from build123d import *

# Parameters (mm, degrees)
SKETCH1_R                  = 1.85
SKETCH1_R_2                = 4
BOSS_EXTRUDE1_DEPTH        = 2
BOSS_EXTRUDE3_DEPTH        = 10
SKETCH12_R                 = 1.36525
CUT_EXTRUDE2_DEPTH         = 3
SKETCH14_R                 = 1.35255
CUT_EXTRUDE3_DEPTH         = 6
FILLET1_R                  = 10
FLATTEN_BENDS1_START       = 2
FLATTEN_BENDS1_DEPTH       = 10
FLATTEN_BENDS1_2_OUTLINE_R = 1.36525
FLATTEN_BENDS1_2_DEPTH     = 2
PROCESS_BENDS1_START       = -8.401979777
PROCESS_BENDS1_OUTLINE_W   = 29
PROCESS_BENDS1_OUTLINE_H   = 2
PROCESS_BENDS1_DEPTH       = 8.701769682
PROCESS_BENDS1_START_2     = 0.591569905
PROCESS_BENDS1_2_OUTLINE_W = 29
PROCESS_BENDS1_2_OUTLINE_H = 10
PROCESS_BENDS1_2_OUTLINE_R = 1.36525
PROCESS_BENDS1_2_DEPTH     = 1.70822
PROCESS_BENDS1_START_3     = 0.299789905
PROCESS_BENDS1_3_OUTLINE_W = 29
PROCESS_BENDS1_3_OUTLINE_H = 10
PROCESS_BENDS1_3_OUTLINE_R = 1.36525
PROCESS_BENDS1_3_DEPTH     = 3
PROCESS_BENDS1_START_4     = -6.292093187
PROCESS_BENDS1_4_DEPTH     = 29


with BuildPart() as part:
    # Sketch1 → Boss-Extrude1 (new body)
    with BuildSketch(Plane(origin=(0, 2, 0), x_dir=(1, 0, 0), z_dir=(0, 1, 0))):
        with BuildLine():
            Line((16.268898369, 15.844931419), (-4.237198285, -4.661165235))
            Line((-4.237198285, -4.661165235), (7.60163648, -16.5))
            Line((7.60163648, -16.5), (48.167251499, -16.5))
            Line((48.167251499, -16.5), (66.344250399, -13.294904666))
            ThreePointArc((66.344250399, -13.294904666), (77.499939542, -0.040402458), (66.423785357, 13.280634945))
            ThreePointArc((66.423785357, 13.280634945), (42.528480772, 15.498562339), (18.613829789, 13.5))
            Line((18.613829789, 13.5), (16.268898369, 15.844931419))
        make_face()
        with Locations(Location((56, 0, 0), (0, 0, 90))):
            Circle(SKETCH1_R, mode=Mode.SUBTRACT)
        with Locations(Location((64, -8, 0), (0, 0, 90))):
            Circle(SKETCH1_R, mode=Mode.SUBTRACT)
        with Locations(Location((72, 0, 0), (0, 0, 90))):
            Circle(SKETCH1_R, mode=Mode.SUBTRACT)
        with Locations(Location((64, 8, 0), (0, 0, 90))):
            Circle(SKETCH1_R, mode=Mode.SUBTRACT)
        with Locations(Location((64, 0, 0), (0, 0, 90))):
            Circle(SKETCH1_R_2, mode=Mode.SUBTRACT)
    extrude(amount=-BOSS_EXTRUDE1_DEPTH)

    # Sketch5 → Boss-Extrude3 (add)
    with BuildSketch(Plane(origin=(0, 2, 0), x_dir=(1, 0, 0), z_dir=(0, 1, 0))):
        Polygon((16.268898369, 15.844931419), (-4.237198285, -4.661165235), (-2.822984723, -6.075378798), (17.683111932, 14.430717857), align=None)
    extrude(amount=BOSS_EXTRUDE3_DEPTH)

    # Sketch12 → Cut-Extrude2 (cut)
    with BuildSketch(Plane(origin=(0.211983475, 0, 0.211983475), x_dir=(-0.7071067811865475, 0, 0.7071067811865477), z_dir=(-0.7071067811865477, 0, -0.7071067811865475))):
        with Locations((-16.207906813, 8)):
            Circle(SKETCH12_R)
        with Locations((-0.207906813, 8)):
            Circle(SKETCH12_R)
    extrude(amount=-CUT_EXTRUDE2_DEPTH, mode=Mode.SUBTRACT)

    # Sketch14 → Cut-Extrude3 (cut)
    with BuildSketch(Plane(origin=(0, 0, 0), x_dir=(1, 0, 0), z_dir=(0, 1, 0))):
        with Locations(Location((39.946755384, 11.867587507, 0), (0, 0, 270))):
            Circle(SKETCH14_R)
    extrude(amount=CUT_EXTRUDE3_DEPTH, mode=Mode.SUBTRACT)

    # Fillet1
    fillet1_edges = [part.edges().sort_by_distance(p)[0] for p in [
        (7.60163648, 1, 16.5),
    ]]
    fillet(fillet1_edges, radius=FILLET1_R)

    # Flatten-Bends1: read off the stored shape, not the designer's step
    # Flatten-Bends1 outline → Flatten-Bends1 (cut)
    with BuildSketch(Plane(origin=(0, 0, 0), x_dir=(1, 0, 0), z_dir=(0, 1, 0)).offset(FLATTEN_BENDS1_START)):
        Polygon((17.683111932, 14.430717857), (16.479779049, 15.634050739), (16.268898369, 15.844931419), (-4.237198285, -4.661165235), (-4.026317605, -4.872045915), (-2.822984722, -6.075378798), align=None)
    extrude(amount=FLATTEN_BENDS1_DEPTH, mode=Mode.SUBTRACT)

    # Flatten-Bends1 2 outline → Flatten-Bends1 2 (add)
    with BuildSketch(Plane(origin=(0, 0, 0), x_dir=(1, 0, 0), z_dir=(0, 1, 0))):
        Polygon((-4.237198285, -4.661165235), (16.268898369, 15.844931419), (10.115818019, 21.99801177), (-10.390278636, 1.491915115), align=None)
        with Locations((-2.965657433, 3.259682068)):
            Circle(FLATTEN_BENDS1_2_OUTLINE_R, mode=Mode.SUBTRACT)
        with Locations((8.348051066, 14.573390567)):
            Circle(FLATTEN_BENDS1_2_OUTLINE_R, mode=Mode.SUBTRACT)
    extrude(amount=FLATTEN_BENDS1_2_DEPTH)

    # Process-Bends1: read off the stored shape, not the designer's step
    # Process-Bends1 outline → Process-Bends1 (cut)
    with BuildSketch(Plane(origin=(0, 0, 0), x_dir=(0.7071067811865471, 0, -0.707106781186548), z_dir=(0.707106781186548, 0, 0.707106781186547)).offset(PROCESS_BENDS1_START)):
        with Locations((8.207906813, 1)):
            Rectangle(PROCESS_BENDS1_OUTLINE_W, PROCESS_BENDS1_OUTLINE_H)
    extrude(amount=PROCESS_BENDS1_DEPTH, mode=Mode.SUBTRACT)

    # Process-Bends1 2 outline → Process-Bends1 2 (add)
    with BuildSketch(Plane(origin=(0, 0, 0), x_dir=(0.7071067811865471, 0, -0.707106781186548), z_dir=(0.707106781186548, 0, 0.707106781186547)).offset(PROCESS_BENDS1_START_2)):
        with Locations((8.207906813, 7)):
            Rectangle(PROCESS_BENDS1_2_OUTLINE_W, PROCESS_BENDS1_2_OUTLINE_H)
        with Locations((0.207906813, 8)):
            Circle(PROCESS_BENDS1_2_OUTLINE_R, mode=Mode.SUBTRACT)
        with Locations((16.207906813, 8)):
            Circle(PROCESS_BENDS1_2_OUTLINE_R, mode=Mode.SUBTRACT)
    extrude(amount=PROCESS_BENDS1_2_DEPTH)

    # Process-Bends1 3 outline → Process-Bends1 3 (add)
    with BuildSketch(Plane(origin=(0, 0, 0), x_dir=(0.7071067811865471, 0, -0.707106781186548), z_dir=(0.707106781186548, 0, 0.707106781186547)).offset(PROCESS_BENDS1_START_3)):
        with Locations((8.207906813, 7)):
            Rectangle(PROCESS_BENDS1_3_OUTLINE_W, PROCESS_BENDS1_3_OUTLINE_H)
        with Locations((0.207906813, 8)):
            Circle(PROCESS_BENDS1_3_OUTLINE_R, mode=Mode.SUBTRACT)
        with Locations((16.207906813, 8)):
            Circle(PROCESS_BENDS1_3_OUTLINE_R, mode=Mode.SUBTRACT)
    extrude(amount=PROCESS_BENDS1_3_DEPTH)

    # Process-Bends1 4 outline → Process-Bends1 4 (cut)
    with BuildSketch(Plane(origin=(0, 0, 0), x_dir=(0.7071067811865474, 0, 0.7071067811865477), z_dir=(0.7071067811865476, 0, -0.7071067811865476)).offset(PROCESS_BENDS1_START_4)):
        with BuildLine():
            ThreePointArc((3.299789905, -2), (2.592683124, -2.292893219), (2.299789905, -3))
            Line((2.299789905, -3), (2.299789905, -12))
            Line((2.299789905, -12), (3.299789905, -12))
            Line((3.299789905, -12), (3.299789905, -2))
        make_face()
        with BuildLine():
            Line((0.299789905, 0), (0.299789905, -3))
            ThreePointArc((0.299789905, -3), (1.178469562, -0.878679657), (3.299789905, 0))
            Line((3.299789905, 0), (0.299789905, 0))
        make_face()
    extrude(amount=PROCESS_BENDS1_4_DEPTH, mode=Mode.SUBTRACT)


solid = part.part
Verification items for the finished model (mm, model axes). A direction names the side the tool comes from. Coordinates: 2 decimals unless noted, no trailing zeros. Loops run counter-clockwise (first coordinate to the right, second up) from the corner with the lowest first, then second, coordinate; pieces in that order, holes last. Notation, with made-up numbers: (-21.5, -40) -> (1.5, -40) arc R29 ccw to (1.5, -7) -> close; hole circle Ø8 at (-31, 49.25). An arc over 180 degrees is marked (long way). Answer as a JSON object with one key per item and string values. Group by question number.
Item 1: Sectioned sample at C-C on y = 11. Record the boundary of the cut face in (x, z).
Item 2: Scan lines: probe 1 along Z at (x, y) = (64, 0.6); probe 2 along X at (y, z) = (0.65, 0); probe 3 along X at (y, z) = (0.75, 0). Record each from-to range of solid material in increasing order.
Item 3: Depth check by flat-ended pin: pin 1 (3 mm diameter, centred on x = 72, z = 0, fed in from -Y); pin 2 (1 mm diameter, centred on y = 8, z = -12, fed in from +X); pin 3 (4 mm diameter, centred on y = 10.5, z = 6.5, fed in from +X); pin 4 (6 mm diameter, centred on x = 56, z = 0, fed in from +Y). Enter the tip coordinate at first touch or a pass-through.
Item 4: Tool access check on faces 1 (the flat face through (37, 2, 0)), 2 (the cylindrical face through (38.626, 0.986, -12.161)). Record the directions out of +Z, -Z, +X, -X, +Y, -Y that give a thin tool (end or side, any length) a straight path to the whole face; none if there is none.
Item 5: Sectioned sample at B-B on x = 63. Record the boundary of the cut face in (y, z), plus the area to 3 significant figures.
Item 6: Mould release check, pull along X, two halves, no side actions. Record for faces 3 (the cylindrical face through (42.865, 1.014, -15.497)), 4 (the flat face through (7.287, 7.437, -4.034)), 5 (the cylindrical face through (6.48, 0.9, -4.84)): +X half, -X half, draft (parallel to the pull), parting line (faces both ways), or undercut.
Item 7: Sectioned sample at A-A on x = 72. Record the boundary of the cut face in (y, z).
Item 8: Sectioned sample at D-D on z = 11. Record the boundary of the cut face in (x, y), plus the area to 3 significant figures.
Evaluation:
{
 "1": {"outline": "(-4.24, 4.66) -> (16.27, -15.84) -> (17.68, -14.43) -> (-2.82, 6.08) -> close"},
 "2": {"probe 1": "z = -13.7 to -9.85, -6.15 to -4, 4 to 6.15, 9.85 to 13.71", "probe 2": "x = 2.03 to 54.15, 57.85 to 60, 68 to 70.15, 73.85 to 77.5", "probe 3": "x = 1.86 to 54.15, 57.85 to 60, 68 to 70.15, 73.85 to 77.5"},
 "3": {"pin 1": "passes through", "pin 2": "stops at x = 15.75", "pin 3": "stops at x = -1.25", "pin 4": "stops at y = 2"},
 "4": {"face 1": "+Z, +X, +Y", "face 2": "+Y, -Y"},
 "5": {"outline": "(0, -13.86) -> (2, -13.86) -> (2, -9.56) -> (0, -9.56) -> close; (0, -6.44) -> (2, -6.44) -> (2, -3.87) -> (0, -3.87) -> close; (0, 3.87) -> (2, 3.87) -> (2, 6.44) -> (0, 6.44) -> close; (0, 9.56) -> (2, 9.56) -> (2, 13.88) -> (0, 13.88) -> close", "area": "27.5 mm²"},
 "6": {"face 3": "undercut", "face 4": "+X half", "face 5": "-X half"},
 "7": {"outline": "(0, -10.87) -> (2, -10.87) -> (2, -1.85) -> (0, -1.85) -> close; (0, 1.85) -> (2, 1.85) -> (2, 10.87) -> (0, 10.87) -> close"},
 "8": {"outline": "(2.1, 0) -> (71.83, 0) -> (71.83, 2) -> (2.1, 2) -> close", "area": "139 mm²"}
}
